from build123d import *

# Parameters (mm, degrees)
ESBO_O1_R                = 20
ESBO_O1_R_2              = 4
RESSALTO_EXTRUS_O3_DEPTH = 5
ESBO_O1_6_R              = 22
ESBO_O1_6_R_2            = 20
RESSALTO_EXTRUS_O4_DEPTH = 10
ESBO_O1_7_R              = 4
RESSALTO_EXTRUS_O5_DEPTH = 2
ESBO_O2_R                = 16
CORTE_EXTRUS_O1_DEPTH    = 60
RESSALTO_EXTRUS_O6_START = 5
ESBO_O3_R                = 4
RESSALTO_EXTRUS_O6_DEPTH = 5


with BuildPart() as part:
    # Esboço1 → Ressalto-extrusão3 (new body)
    with BuildSketch(Plane.XY):
        Circle(ESBO_O1_R)
        Circle(ESBO_O1_R_2, mode=Mode.SUBTRACT)
    extrude(amount=RESSALTO_EXTRUS_O3_DEPTH)

    # Esboço1<6> → Ressalto-extrusão4 (add)
    with BuildSketch(Plane.XY):
        Circle(ESBO_O1_6_R)
        Circle(ESBO_O1_6_R_2, mode=Mode.SUBTRACT)
    extrude(amount=RESSALTO_EXTRUS_O4_DEPTH)

    # Esboço1<7> → Ressalto-extrusão5 (add)
    with BuildSketch(Plane.XY):
        Circle(ESBO_O1_7_R)
    extrude(amount=RESSALTO_EXTRUS_O5_DEPTH)

    # Esboço2 → Corte-extrusão1 (cut)
    with BuildSketch(Plane.XY.offset(5)):
        Circle(ESBO_O2_R)
    extrude(amount=-CORTE_EXTRUS_O1_DEPTH, mode=Mode.SUBTRACT)

    # Esboço3 → Ressalto-extrusão6 (add)
    with BuildSketch(Plane.XY.offset(RESSALTO_EXTRUS_O6_START)):
        with BuildLine():
            Line((2, -15.874507866), (2, -5.656854249))
            ThreePointArc((2, -5.656854249), (4.243647898, -4.241633237), (5.657803332, -1.997313561))
            Line((5.657803332, -1.997313561), (15.874846095, -1.997313561))
            ThreePointArc((15.874846095, -1.997313561), (16, 0), (15.874846095, 1.997313561))
            Line((15.874846095, 1.997313561), (5.657803332, 1.997313561))
            ThreePointArc((5.657803332, 1.997313561), (4.243647898, 4.241633237), (2, 5.656854249))
            Line((2, 5.656854249), (2, 15.874507866))
            ThreePointArc((2, 15.874507866), (0, 16), (-2, 15.874507866))
            Line((-2, 15.874507866), (-2, 5.656854249))
            ThreePointArc((-2, 5.656854249), (-4.243647898, 4.241633237), (-5.657803332, 1.997313561))
            Line((-5.657803332, 1.997313561), (-15.874846095, 1.997313561))
            ThreePointArc((-15.874846095, 1.997313561), (-16, 0), (-15.874846095, -1.997313561))
            Line((-15.874846095, -1.997313561), (-5.657803332, -1.997313561))
            ThreePointArc((-5.657803332, -1.997313561), (-4.243647898, -4.241633237), (-2, -5.656854249))
            Line((-2, -5.656854249), (-2, -15.874507866))
            ThreePointArc((-2, -15.874507866), (0, -16), (2, -15.874507866))
        make_face()
        Circle(ESBO_O3_R, mode=Mode.SUBTRACT)
    extrude(amount=-RESSALTO_EXTRUS_O6_DEPTH)


solid = part.part
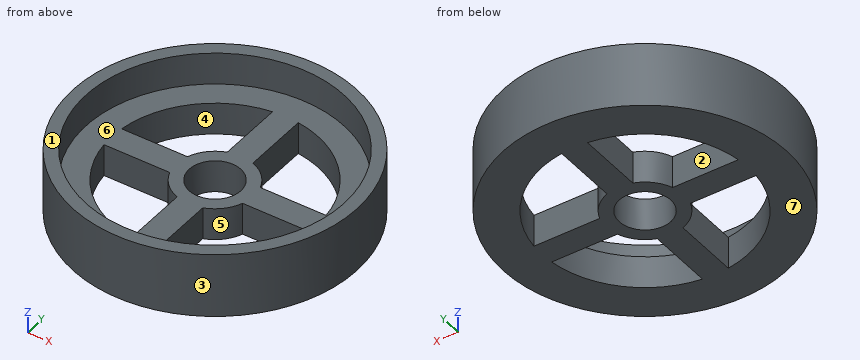
Input: part model. Units: mm. Frame: model coordinates. Face numbers are marked on the shaded views. A direction names the side the tool comes from. Round coordinates to 2 decimals unless told otherwise and drop trailing zeros. Loops run counter-clockwise (first coordinate to the right, second up) from the corner with the lowest first, then second, coordinate; pieces in that order, holes last. Notation, with made-up numbers: (12.5, -39) -> (59.5, -39) arc R27 ccw to (59.5, -20) -> close; hole circle Ø1 at (87, 34.5). An arc over 180 degrees is marked (long way). Answer as a JSON object with one key per item and string values. Group by question number.
1) Section query A-A on y = 0. Output: boundary loops of the cut face in (x, z), plus the area to 3 significant figures.
2) Reachability of the marked faces 5, 6 and 7 from +Z, -Z, +X, -X, +Y, -Y: full face, straight path, thin tool, end or side. Return the list, or none.
3) Draft query along X for the marked faces 1, 2, 3 and 4. Return one class per face: +X half, -X half, draft (parallel to the pull), parting line (faces both ways), or undercut.
4) Section query C-C on z = 2.75. Output: boundary loops of the cut face in (x, y), plus the area to 3 significant figures.
5) Pin query (flat end, axial travel): pin 1 (1 mm diameter, centred on x = 0.5, z = 1.5, fed in from +Y); pin 2 (1 mm diameter, centred on x = 8.5, z = 3.5, fed in from -Y); pin 3 (5.5 mm diameter, centred on y = -11, z = 2.5, fed in from +X). Return the tip coordinate at first contact, or that it passes through.
6) Section query D-D on y = -7. Output: boundary loops of the cut face in (x, z) (1 decimal).
7) Ray query, L1, parallel to Y at x = 7.5, z = 2.5; L2, parallel to Y at x = 0, z = 8; L3, parallel to Y at x = 0, z = 3.6. Return the intervals inside material, ascending.
Reply:
{
 "1": {"outline": "(-22, 0) -> (-4, 0) -> (-4, 5) -> (-20, 5) -> (-20, 10) -> (-22, 10) -> close; (4, 0) -> (22, 0) -> (22, 10) -> (20, 10) -> (20, 5) -> (4, 5) -> close", "area": "200 mm2"},
 "2": {"face 5": "+Z, -Z", "face 6": "+Z", "face 7": "-Z, +X, -X, +Y, -Y"},
 "3": {"face 1": "draft", "face 2": "undercut", "face 3": "parting line", "face 4": "undercut"},
 "4": {"outline": "circle Ø44 at (0, 0); hole (-15.87, -2) arc R16 ccw to (-2, -15.87) -> (-2, -5.66) arc R6 cw to (-5.66, -2) -> close; hole (-15.87, 2) -> (-5.66, 2) arc R6 cw to (-2, 5.66) -> (-2, 15.87) arc R16 ccw to start; hole circle Ø8 at (0, 0); hole (2, -15.87) arc R16 ccw to (15.87, -2) -> (5.66, -2) arc R6 cw to (2, -5.66) -> close; hole (2, 5.66) arc R6 cw to (5.66, 2) -> (15.87, 2) arc R16 ccw to (2, 15.87) -> close", "area": "940 mm2"},
 "5": {"pin 1": "stops at y = 22", "pin 2": "stops at y = -20.49", "pin 3": "stops at x = 20.39"},
 "6": {"outline": "(-20.9, 0) -> (-14.4, 0) -> (-14.4, 5) -> (-18.7, 5) -> (-18.7, 10) -> (-20.9, 10) -> close; (-2, 0) -> (2, 0) -> (2, 5) -> (-2, 5) -> close; (14.4, 0) -> (20.9, 0) -> (20.9, 10) -> (18.7, 10) -> (18.7, 5) -> (14.4, 5) -> close"},
 "7": {"L1": "y = -20.68 to -14.13, -2 to 2, 14.13 to 20.68", "L2": "y = -22 to -20, 20 to 22", "L3": "y = -22 to -4, 4 to 22"}
}
